Verification items for the finished model (mm, model axes). A direction names the side the tool comes from. Give positions to 0.01 mm unless a question says otherwise; leave off trailing zeros. Loops run counter-clockwise (first coordinate to the right, second up) from the corner with the lowest first, then second, coordinate; pieces in that order, holes last. Notation, with made-up numbers: (70.25, -6.75) - (119.25, -6.75) arc R9 ccw to (119.25, 7.25) - close; hole circle Ø8 at (53.25, 30.5). An arc over 180 degrees is marked (long way). Answer in a Markdown table with one row per item.
```python
from build123d import *

# Parameters (mm, degrees)
SKETCH006_W     = 210
SKETCH006_H     = 70
PAD002_DEPTH    = 68
POCKET_DEPTH    = 65
SKETCH_W        = 7
SKETCH_H        = 5
POCKET001_DEPTH = 20
SKETCH008_W     = 6
SKETCH008_H     = 6
POCKET002_DEPTH = 10


with BuildPart() as part:
    # Sketch006 → Pad002 (new body)
    with BuildSketch(Plane.XY):
        with Locations((28.778721, -0.538714)):
            Rectangle(SKETCH006_W, SKETCH006_H)
    extrude(amount=PAD002_DEPTH)

    # Sketch007 (on Face5 of Pad002) → Pocket (cut)
    with BuildSketch(Plane(origin=(0, 0, 0), x_dir=(1, 0, 0), z_dir=(0, 0, -1))):
        Polygon((-66.221279, 31.538714), (-66.221279, 25.538714), (-72.221279, 25.538714), (-72.221279, -24.461286), (-66.221279, -24.461286), (-66.221279, -30.461286), (123.778721, -30.461286), (123.778721, -24.461286), (129.778721, -24.461286), (129.778721, 25.538714), (123.778721, 25.538714), (123.778721, 31.538714), align=None)
    extrude(amount=-POCKET_DEPTH, mode=Mode.SUBTRACT)

    # Sketch (on Face4 of Pad002) → Pocket001 (cut)
    with BuildSketch(Plane(origin=(-76.221279, 0, 0), x_dir=(0, -1, 0), z_dir=(-1, 0, 0))):
        with Locations((-13.5, 32.5)):
            Rectangle(SKETCH_W, SKETCH_H)
        with Locations((13.5, 32.5)):
            Rectangle(SKETCH_W, SKETCH_H)
    extrude(amount=-POCKET001_DEPTH, mode=Mode.SUBTRACT)

    # Sketch008 (on Face2 of Pad002) → Pocket002 (cut)
    with BuildSketch(Plane.YZ.offset(133.778721)):
        with Locations((0, 3)):
            Rectangle(SKETCH008_W, SKETCH008_H)
    extrude(amount=-POCKET002_DEPTH, mode=Mode.SUBTRACT)


solid = part.part
```
Q1. Draft check along X on faces 1 (the face through (-66.221, -29, 32)), 2 (the face through (-76.221, -1, 34)), 3 (the face through (-74, -13, 30)). Enter one of: +X half, -X half, draft (parallel to the pull), parting line (faces both ways), or undercut.
Completed:
| item | result |
|---|---|
| face 1 | undercut |
| face 2 | -X half |
| face 3 | draft |
Q2. Thickness scan on line 1 (Y direction, x = -40.5, z = 35); line 2 (X direction, y = -6, z = 63.5); line 3 (X direction, y = 27, z = 30). Record the ranges inside material, lowest first.
Completed:
| item | result |
|---|---|
| line 1 | -35.54 to -31.54, 30.46 to 34.46 |
| line 2 | -76.22 to -72.22, 129.78 to 133.78 |
| line 3 | -76.22 to -66.22, 123.78 to 133.78 |
Q3. Sectioned sample at C-C (x = 5). Record the cut outline in (y, z), and give its area (3 significant figures).
Completed:
| item | result |
|---|---|
| outline | (-35.54, 0) - (-31.54, 0) - (-31.54, 65) - (30.46, 65) - (30.46, 0) - (34.46, 0) - (34.46, 68) - (-35.54, 68) - close |
| area | 730 mm^2 |
Q4. Sectioned sample at D-D (y = -0.5). Record the cut outline in (x, z).
Completed:
| item | result |
|---|---|
| outline | (-76.22, 0) - (-72.22, 0) - (-72.22, 65) - (129.78, 65) - (129.78, 6) - (133.78, 6) - (133.78, 68) - (-76.22, 68) - close |
Q5. Sectioned sample at A-A (y = -15). Record the cut outline in (x, z).
Completed:
| item | result |
|---|---|
| outline | (-76.22, 0) - (-72.22, 0) - (-72.22, 30) - (-76.22, 30) - close; (-76.22, 35) - (-72.22, 35) - (-72.22, 65) - (129.78, 65) - (129.78, 0) - (133.78, 0) - (133.78, 68) - (-76.22, 68) - close |
Q6. Go/stop test with flat-tipped pins: P1, Ø2, axis at x = 132.5, y = 0.5, coming from the -Z side; P2, Ø5, axis at x = -6, y = -7, coming from the -Z side. Record where each tip stops, or that it passes through.
Completed:
| item | result |
|---|---|
| P1 | z = 6 |
| P2 | z = 65 |
Q7. Tool access check on faces 4 (the face through (132, -3, 3)), 5 (the face through (-66.221, 27, 32)), 6 (the face through (-74, -10, 32)). Record the directions out of +Z, -Z, +X, -X, +Y, -Y that give a thin tool (end or side, any length) a straight path to the whole face; none if there is none.
Completed:
| item | result |
|---|---|
| face 4 | -Z, +X |
| face 5 | -Z |
| face 6 | -X |
Q8. Sectioned sample at B-B (z = 51). Record the cut outline in (x, y), and give its area (3 significant figures).
Completed:
| item | result |
|---|---|
| outline | (-76.22, -35.54) - (133.78, -35.54) - (133.78, 34.46) - (-76.22, 34.46) - close; hole (-72.22, -25.54) - (-66.22, -25.54) - (-66.22, -31.54) - (123.78, -31.54) - (123.78, -25.54) - (129.78, -25.54) - (129.78, 24.46) - (123.78, 24.46) - (123.78, 30.46) - (-66.22, 30.46) - (-66.22, 24.46) - (-72.22, 24.46) - close |
| area | 2,320 mm^2 |
